Part model, mm, in its own coordinate system. Face numbers are marked on the shaded views. A direction names the side the tool comes from. Coordinates: 2 decimals unless noted, no trailing zeros. Write each loop counter-clockwise with the first axis right and the second up, starting at its lowest first coordinate (ties: lowest second). Pieces come first, ordered by that corner, then holes. Notation, with made-up numbers: (66.5, 82) - (95.5, 82) arc R20 ccw to (95.5, 108) - close; hole circle Ø7 at (18, -10.5). An arc over 180 degrees is marked (long way). Use one line per item in the form item = value. Start each with the question number.
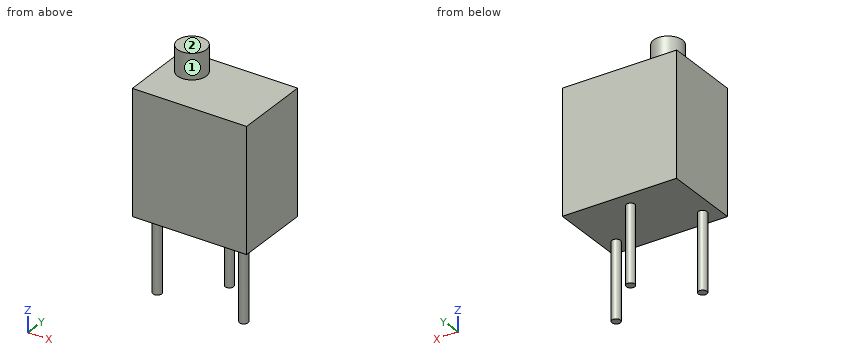
from build123d import *

# Parameters (mm, degrees)
EXTRUDE_1_DEPTH      = 2.25
EXTRUDE_1_DEPTH_BACK = 2.25
SKETCH_1_W           = 6.71
SKETCH_1_H           = 7.24
SKETCH_3_R           = 0.25
EXTRUDE_3_DEPTH      = 4.5
SKETCH_4_R           = 0.85
EXTRUDE_4_DEPTH      = 1.5


with BuildPart() as part:
    # Sketch 1 → Extrude 1 (new, two sides: drawn at the far end of the back side and taken through both)
    with BuildSketch(Plane(origin=(0, 0, 0), x_dir=(1, 0, 0), z_dir=(0, 1, 0)).offset(-EXTRUDE_1_DEPTH_BACK)):
        Rectangle(SKETCH_1_W, SKETCH_1_H)
    extrude(amount=EXTRUDE_1_DEPTH + EXTRUDE_1_DEPTH_BACK)

    # Sketch 3 → Extrude 3 (add)
    with BuildSketch(Plane(origin=(0, 0, -3.62), x_dir=(-1, 0, 0), z_dir=(0, 0, -1))):
        with Locations(Location((0, 1.27, 0), (0, 0, 180))):
            Circle(SKETCH_3_R)
        with Locations(Location((2.54, -1.27, 0), (0, 0, 180))):
            Circle(SKETCH_3_R)
        with Locations(Location((-2.54, -1.27, 0), (0, 0, 180))):
            Circle(SKETCH_3_R)
    extrude(amount=EXTRUDE_3_DEPTH)

    # Sketch 4 → Extrude 4 (add)
    with BuildSketch(Plane.XY.offset(3.62)):
        with Locations(Location((-1.855, 0.75, 0), (0, 0, 180))):
            Circle(SKETCH_4_R)
    extrude(amount=EXTRUDE_4_DEPTH)


solid = part.part
Q1. Slice it at B-B (x = -2.54). List the corners of the cut face in (y, z).
Q2. Slice it at C-C (z = -6.75). List the corners of the cut face in (x, y).
Q3. Pin check, flat tips, straight feed: P1, Ø1, axis at y = -1, z = -5, coming from the -X side; P2, Ø2, axis at x = 1.5, y = -0.5, coming from the +Z side; P3, Ø2, axis at x = -2.5, z = -6, coming from the -Y side. Stop position of each tip, or through.
Q4. Slice it at A-A (y = -1.27). List the corners of the cut face in (x, z) (3 decimals).
Q5. Which spindle directions (+Z, -Z, +X, -X, +Y, -Y) get a long thin tool onto all of the face, cutting with end or side? Do the marked faces 1 and 2. Say none if no direction does.
Q6. Slice it at D-D (y = 0.75). List the corners of the cut face in (x, z) (3 decimals), plus the area to 3 significant figures.
Q7. Drill centre lines: probe 1 along Z at (x, y) = (2, -1.45); probe 2 along Z at (x, y) = (-2.5, 0.7); probe 3 along X at (y, z) = (-1.45, -5.5). Where is each one in solid material? Low to high.
Solution:
q1.outline = (-2.25, -3.62) - (-1.52, -3.62) - (-1.52, -8.12) - (-1.02, -8.12) - (-1.02, -3.62) - (2.25, -3.62) - (2.25, 3.62) - (1.25, 3.62) - (1.25, 5.12) - (0.25, 5.12) - (0.25, 3.62) - (-2.25, 3.62) - close
q2.outline = circle Ø0.5 at (-2.54, -1.27); circle Ø0.5 at (0, 1.27); circle Ø0.5 at (2.54, -1.27)
q3.P1 = -2.79
q3.P2 = 3.62
q3.P3 = -1.52
q4.outline = (-3.355, -3.62) - (-2.79, -3.62) - (-2.79, -8.12) - (-2.29, -8.12) - (-2.29, -3.62) - (2.29, -3.62) - (2.29, -8.12) - (2.79, -8.12) - (2.79, -3.62) - (3.355, -3.62) - (3.355, 3.62) - (-3.355, 3.62) - close
q5.face_1 = +Z
q5.face_2 = +Z, +X, -X, +Y, -Y
q6.outline = (-3.355, -3.62) - (3.355, -3.62) - (3.355, 3.62) - (-1.005, 3.62) - (-1.005, 5.12) - (-2.705, 5.12) - (-2.705, 3.62) - (-3.355, 3.62) - close
q6.area = 51.1 mm2
q7.probe_1 = -3.62 to 3.62
q7.probe_2 = -3.62 to 5.12
q7.probe_3 = -2.71 to -2.37, 2.37 to 2.71
